from build123d import *

# Parameters (mm, degrees)
F0_W     = 3.2
F0_H     = 12
F0_R     = 1.65
F0_H_2   = 6
F0_W_2   = 50
F0_H_3   = 3
F0_W_3   = 20
F1_DEPTH = 3


with BuildPart() as f1:
    # F0 (on Front) → F1 (new body)
    with BuildSketch(Plane.XZ):
        Polygon((70, -25), (85, -25), (85, 25), (25, 25), (-25, 25), (-85, 25), (-85, -25), (-70, -25), (-50, -25), (-30, -25), (-10, -25), (10, -25), (30, -25), (50, -25), align=None)
        with Locations((-79.4, -15)):
            Rectangle(F0_W, F0_H, mode=Mode.SUBTRACT)
        with Locations((79.4, -15)):
            Rectangle(F0_W, F0_H, mode=Mode.SUBTRACT)
        with Locations((-79.4, 0)):
            Circle(F0_R, mode=Mode.SUBTRACT)
        with Locations((-79.4, 16)):
            Rectangle(F0_W, F0_H_2, mode=Mode.SUBTRACT)
        with Locations((79.4, 0)):
            Circle(F0_R, mode=Mode.SUBTRACT)
        with Locations((79.4, 16)):
            Rectangle(F0_W, F0_H_2, mode=Mode.SUBTRACT)
        with Locations((0, 26.5)):
            Rectangle(F0_W_2, F0_H_3)
        with Locations((-60, -26.5)):
            Rectangle(F0_W_3, F0_H_3)
        with Locations((-20, -26.5)):
            Rectangle(F0_W_3, F0_H_3)
        with Locations((20, -26.5)):
            Rectangle(F0_W_3, F0_H_3)
        with Locations((60, -26.5)):
            Rectangle(F0_W_3, F0_H_3)
    extrude(amount=F1_DEPTH)


solid = f1.part
Check sheet for the modelled part. Datum: model origin and axes. Units: mm. A direction names the side the tool comes from. Give positions to 0.01 mm unless a question says otherwise; leave off trailing zeros. Order: outer loops, then holes, each group sorted by start corner. A loop starts at its lowest first (then second) coordinate and runs counter-clockwise, first axis right, second up. Notation, with made-up numbers: M 79.5,10.25 L 122.5,10.25 A7 ccw 122.5,21.25 Z; hole C -31.75,-21 d1. An arc over 180 degrees is marked long. Answer as CSV lines item,"result". Start each with the question number.
Item 1: Tool access check on faces 1 (the face through (81, -1, 16)), 2 (the face through (25, -1, 26)), 3 (the face through (0, -1, -25)). Record the directions out of +Z, -Z, +X, -X, +Y, -Y that give a thin tool (end or side, any length) a straight path to the whole face; none if there is none.
Item 2: Gauge pin test, flat ends, axial feed: P1, Ø0.9, axis at x = -36.5, y = -1, coming from the -Z side; P2, Ø0.9, axis at x = 79, y = -1.5, coming from the +Z side; P3, Ø0.9, axis at y = -1.5, z = 26, coming from the -X side. Record the tip position at first contact, or that the pin passes through.
Item 3: Cross-section at A-A on x = -79.4. Enter the section's corners in (y, z).
Item 4: Cross-section at C-C on x = 4. Enter the section's corners in (y, z).
Item 5: Cross-section at B-B on y = -1. State how many separate pieces and enclosed holes the cut face has, plus the area to 3 significant figures.
Item 6: Mould release check, pull along Z, two halves, no side actions. Record for faces 4 (the face through (-25, -1, 26)), 5 (the face through (-79, -1, 19)), 6 (the face through (20, -1, -28)): +Z half, -Z half, draft (parallel to the pull), parting line (faces both ways), or undercut.
Item 7: Thickness scan on line 1 (X direction, y = -1.4, z = 17); line 2 (Z direction, x = 79.4, y = -1.55); line 3 (Z direction, x = -41.5, y = -1.1). Record the ranges inside material, lowest first. Write a range as [from, to].
Established:
1,face 1,"+Y, -Y"
1,face 2,"+Z, +X, +Y, -Y"
1,face 3,"-Z, +Y, -Y"
2,P1,"stops at z = -25"
2,P2,"stops at z = 25"
2,P3,"stops at x = -25"
3,outline,"M -3,-25 L 0,-25 L 0,-21 L -3,-21 Z; M -3,-9 L 0,-9 L 0,-1.65 L -3,-1.65 Z; M -3,1.65 L 0,1.65 L 0,13 L -3,13 Z; M -3,19 L 0,19 L 0,25 L -3,25 Z"
4,outline,"M -3,-25 L 0,-25 L 0,28 L -3,28 Z"
5,separate pieces,"1"
5,enclosed holes,"6"
5,area,"8,760 mm^2"
6,face 4,"draft"
6,face 5,"undercut"
6,face 6,"-Z half"
7,line 1,"x = [-85, -81], [-77.8, 77.8], [81, 85]"
7,line 2,"z = [-25, -21], [-9, -1.65], [1.65, 13], [19, 25]"
7,line 3,"z = [-25, 25]"
